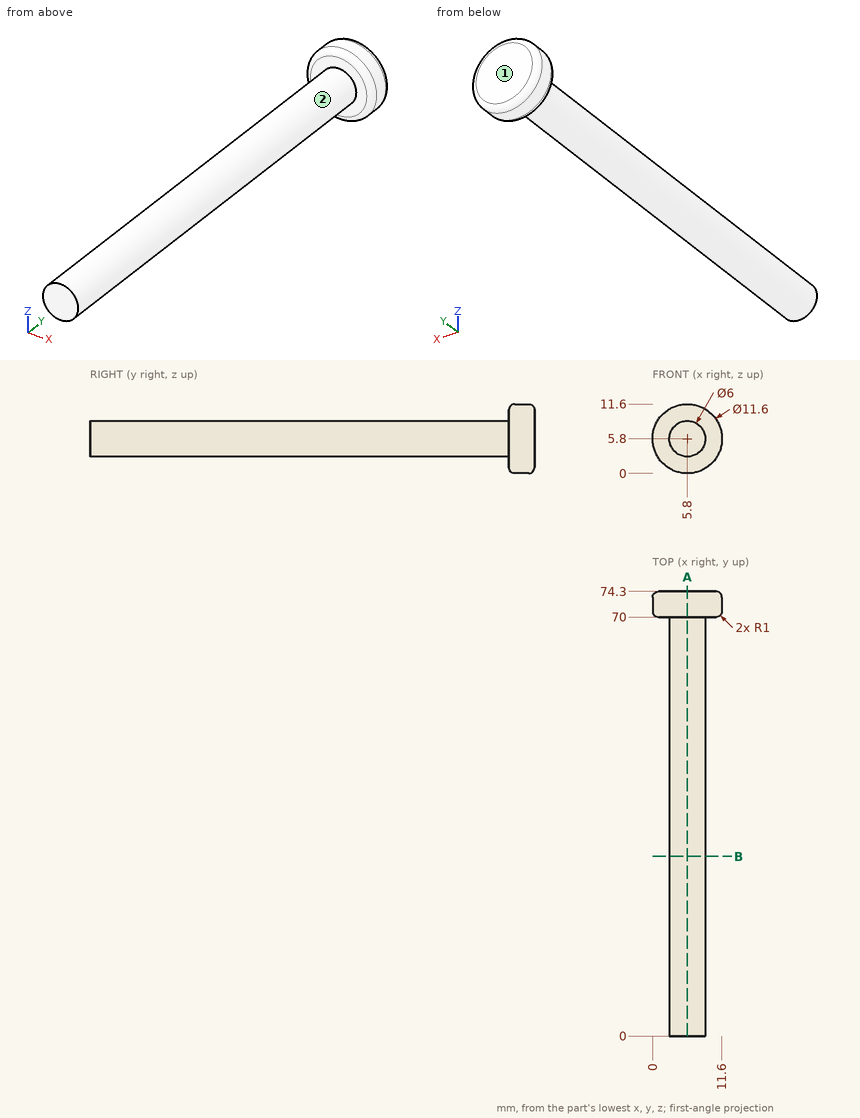
Job drawing, mm, ordinate dimensions from the low corner. One solid piece. A direction names the side the tool comes from. Round coordinates to 2 decimals unless told otherwise and drop trailing zeros. Loops run counter-clockwise (first coordinate to the right, second up) from the corner with the lowest first, then second, coordinate; pieces in that order, holes last. Notation, with made-up numbers: (43, -11) -> (53, -11) arc R25 ccw to (53, 28) -> close; hole circle Ø9 at (-37.5, 28). An arc over 180 degrees is marked (long way). Use a Markdown table: item, result.
1) Cut at A-A, the plane x = 5.8. List the corners of the cut face in (y, z), and give its area (3 significant figures).
The answers:
| item | result |
|---|---|
| outline | (0, 2.8) -> (70, 2.8) -> (70, 1) arc R1 ccw to (71, 0) -> (73.3, 0) arc R1 ccw to (74.3, 1) -> (74.3, 10.6) arc R1 ccw to (73.3, 11.6) -> (71, 11.6) arc R1 ccw to (70, 10.6) -> (70, 8.8) -> (0, 8.8) -> close |
| area | 469 mm2 |
2) Tool access for the marked faces 1 and 2: list every direction of +Z, -Z, +X, -X, +Y, -Y with a clear straight run to the whole face (end or side of a thin tool).
The answers:
| item | result |
|---|---|
| face 1 | +Z, -Z, +X, -X, +Y |
| face 2 | -Y |
3) Cut at B-B, the plane y = 30. List the corners of the cut face in (x, z), and give its area (3 significant figures).
The answers:
| item | result |
|---|---|
| outline | circle Ø6 at (5.8, 5.8) |
| area | 28.3 mm2 |
4) Probe line 1 (Y direction, x = 10.25, z = 5.5); line 2 (Z direction, x = 5.5, y = 67.5); line 3 (Z direction, x = 4, y = 7). List the from-to ranges inside material, lowest first. Write a range as [from, to].
The answers:
| item | result |
|---|---|
| line 1 | y = [70, 74.3] |
| line 2 | z = [2.82, 8.78] |
| line 3 | z = [3.4, 8.2] |
5) Drop flat-ended pins along their axis: pin 1 Ø1.5 at (x, y) = (6.5, 52) entering from -Z; pin 2 Ø2 at (y, z) = (22.5, 3) entering from -X; pin 3 Ø1 at (x, y) = (7, 22) entering from +Z. Give the stop position or say it passes through.
The answers:
| item | result |
|---|---|
| pin 1 | stops at z = 2.8 |
| pin 2 | stops at x = 3.4 |
| pin 3 | stops at z = 8.72 |
